```python
from build123d import *

# Parameters (mm, degrees)
F0_W           = 109.5375
F0_H           = 109.5375
F0_W_2         = 11.1125
F0_H_2         = 23.8125
F0_W_3         = 10.31875
F1_DEPTH       = 6.35
F1_TAPER       = -26.565
F2_D           = 3.175
F2_DEPTH       = 9.525
F2_CSINK_D     = 6.35
F2_CSINK_ANGLE = 90
F2_TIP         = 0.9538662327
F3_D           = 3.175
F3_DEPTH       = 9.525
F3_CSINK_D     = 6.35
F3_CSINK_ANGLE = 90
F3_TIP         = 0.9538662327
F4_D           = 3.175
F4_DEPTH       = 9.525
F4_CSINK_D     = 6.35
F4_CSINK_ANGLE = 90
F4_TIP         = 0.9538662327
F5_D           = 3.175
F5_DEPTH       = 9.525
F5_CSINK_D     = 6.35
F5_CSINK_ANGLE = 90
F5_TIP         = 0.9538662327
F6_R           = 6.35
F7_W           = 111.125
F7_H           = 111.125
F7_R           = 1.5875
F7_W_2         = 4.7625141797
F7_H_2         = 17.4625141797
F7_W_3         = 3.9687641797
F8_DEPTH       = 3.175
F8_TAPER       = 25


with BuildPart() as f1:
    # F0 (on Front) → F1 (new body)
    with BuildSketch(Plane.XZ):
        with Locations((0.79375, 3.095625)):
            Rectangle(F0_W, F0_H)
        with Locations((-21.828125, 1.905)):
            Rectangle(F0_W_2, F0_H_2, mode=Mode.SUBTRACT)
        with Locations((23.8125, 1.905)):
            Rectangle(F0_W_3, F0_H_2, mode=Mode.SUBTRACT)
    extrude(amount=F1_DEPTH, taper=F1_TAPER)

    # F2
    with Locations(Plane(origin=(0, 0, 0), x_dir=(1, 0, 0), z_dir=(0, 1, 0))):
        with Locations((-21.828125, -31.670625)):
            CounterSinkHole(F2_D / 2, F2_CSINK_D / 2, depth=F2_DEPTH, counter_sink_angle=F2_CSINK_ANGLE)
            with Locations((0, 0, -(F2_DEPTH + F2_TIP / 2))):  # 118° drill point
                Cone(0, F2_D / 2, F2_TIP, mode=Mode.SUBTRACT)

    # F3
    with Locations(Plane(origin=(0, 0, 0), x_dir=(1, 0, 0), z_dir=(0, 1, 0))):
        with Locations((23.415625, -31.670625)):
            CounterSinkHole(F3_D / 2, F3_CSINK_D / 2, depth=F3_DEPTH, counter_sink_angle=F3_CSINK_ANGLE)
            with Locations((0, 0, -(F3_DEPTH + F3_TIP / 2))):  # 118° drill point
                Cone(0, F3_D / 2, F3_TIP, mode=Mode.SUBTRACT)

    # F4
    with Locations(Plane(origin=(0, 0, 0), x_dir=(1, 0, 0), z_dir=(0, 1, 0))):
        with Locations((23.415625, 27.860625)):
            CounterSinkHole(F4_D / 2, F4_CSINK_D / 2, depth=F4_DEPTH, counter_sink_angle=F4_CSINK_ANGLE)
            with Locations((0, 0, -(F4_DEPTH + F4_TIP / 2))):  # 118° drill point
                Cone(0, F4_D / 2, F4_TIP, mode=Mode.SUBTRACT)

    # F5
    with Locations(Plane(origin=(0, 0, 0), x_dir=(1, 0, 0), z_dir=(0, 1, 0))):
        with Locations((-21.828125, 27.860625)):
            CounterSinkHole(F5_D / 2, F5_CSINK_D / 2, depth=F5_DEPTH, counter_sink_angle=F5_CSINK_ANGLE)
            with Locations((0, 0, -(F5_DEPTH + F5_TIP / 2))):  # 118° drill point
                Cone(0, F5_D / 2, F5_TIP, mode=Mode.SUBTRACT)

    # F6
    f6_edges = [f1.edges().sort_by_distance(p)[0] for p in [
        (0.79375, 0, 57.864375),
        (55.5625, 0, 3.095625),
        (-53.975, 0, 3.095625),
        (0.79375, 0, -51.673125),
    ]]
    fillet(f6_edges, radius=F6_R)

    # F7 (on face) → F8 (cut)
    with BuildSketch(Plane.XZ.offset(6.35)):
        with Locations((0.79375, 3.095625)):
            Rectangle(F7_W, F7_H)
        with Locations((-21.828125, -27.860625)):
            Circle(F7_R, mode=Mode.SUBTRACT)
        with Locations((-21.828125, 1.905)):
            Rectangle(F7_W_2, F7_H_2, mode=Mode.SUBTRACT)
        with Locations((23.415625, -27.860625)):
            Circle(F7_R, mode=Mode.SUBTRACT)
        with Locations((23.8125, 1.905)):
            Rectangle(F7_W_3, F7_H_2, mode=Mode.SUBTRACT)
        with Locations((-21.828125, 31.670625)):
            Circle(F7_R, mode=Mode.SUBTRACT)
        with Locations((23.415625, 31.670625)):
            Circle(F7_R, mode=Mode.SUBTRACT)
    extrude(amount=-F8_DEPTH, taper=F8_TAPER, mode=Mode.SUBTRACT)


solid = f1.part
```
Source: CAD feature listing. Evaluate the final solid. Frame: model axes, mm. A direction names the side the tool comes from. Give positions to 0.01 mm unless a question says otherwise; leave off trailing zeros. Use a Markdown table: item, result.
Q1. Material intervals for line 1 (X direction, y = -1.5, z = -2); line 2 (X direction, y = -3, z = 12); line 3 (Y direction, x = 22, z = 51) (3 decimals), sorted ascending. Write a range as [from, to].
A:
| item | result |
|---|---|
| line 1 | [-54.15, -26.63], [-17.02, 19.4], [28.22, 55.74] |
| line 2 | [-55.44, -25.88], [-17.77, 20.15], [27.47, 57.03] |
| line 3 | [-3.175, 0] |
Q2. First-contact query: P1, Ø2, axis at x = 39, y = -3.5, coming from the +Z side; P2, Ø3, axis at x = -21.83, z = 31.67, coming from the +Y side; P3, Ø1.5, axis at x = 27.5, y = -1.5, coming from the -Z side; P4, Ø6, axis at x = 1.5, z = -23, coming from the -Y side (3 decimals). Flat tips, straight axial feed; report the tip coordinate or a pass-through.
A:
| item | result |
|---|---|
| P1 | z = 60.11 |
| P2 | through |
| P3 | z = -52.6 |
| P4 | y = -3.175 |
Q3. Pull-direction query (Z, two-part tool) for faces 1 (the face through (23.76, -4, 33.22)), 2 (the face through (-22.56, -4, -26.45)), 3 (the face through (-1, 0, 3)); classes: +Z half, -Z half, draft (parallel to the pull), parting line (faces both ways), or undercut.
A:
| item | result |
|---|---|
| face 1 | undercut |
| face 2 | undercut |
| face 3 | draft |
Q4. Section A-A (z = -1.5). State how many separate pieces and enclosed holes the cut face has, and give its area (3 significant figures).
A:
| item | result |
|---|---|
| separate pieces | 3 |
| enclosed holes | 0 |
| area | 304 mm^2 |
Q5. Access query for faces 4 (the face through (-56, -6.35, -1)), 5 (the face through (-1, -3.175, 3)). Directions: +Z, -Z, +X, -X, +Y, -Y. A direction counts if a zero-diameter tool reaches every point of the face in a straight line with its end or side. Return the directions, or none.
A:
| item | result |
|---|---|
| face 4 | +Z, -Z, +X, -X, -Y |
| face 5 | -Y |
